Work out the finished part from the listing and answer in its coordinate system (mm). Coordinates: 2 decimals unless noted, no trailing zeros. Loops run counter-clockwise (first coordinate to the right, second up) from the corner with the lowest first, then second, coordinate; pieces in that order, holes last. Notation, with made-up numbers: (59, 63) -> (65, 63) arc R19 cw to (65, 69) -> close; hole circle Ø9 at (-0.75, 3). An arc over 180 degrees is marked (long way). One line per question, with ' | ' between items.
```python
from build123d import *

# Parameters (mm, degrees)
SKETCH_1_R      = 1.5
SKETCH_1_R_2    = 1.785756588
SKETCH_1_R_3    = 1.689732538
EXTRUDE_1_DEPTH = 6


with BuildPart() as part:
    # 草图1 → 凸台-拉伸1 (new body)
    # profile 1 of 2: a face of its own
    with BuildSketch(Plane(origin=(0, 0, 0), x_dir=(0, 0, -1), z_dir=(1, 0, 0))):
        with BuildLine():
            ThreePointArc((-172.5, 0), (0, -172.5), (172.5, 0))
            Line((172.5, 0), (-41.730591699, 0))
            Line((-41.730591699, 0), (-41.730591699, -2))
            ThreePointArc((-41.730591699, -2), (-42.023484918, -2.707106781), (-42.730591699, -3))
            Line((-42.730591699, -3), (-80.730591699, -3))
            ThreePointArc((-80.730591699, -3), (-81.43769848, -2.707106781), (-81.730591699, -2))
            Line((-81.730591699, -2), (-81.730591699, 0))
            Line((-81.730591699, 0), (-172.5, 0))
        make_face()
        with Locations((-138.564064605, -80)):
            Circle(SKETCH_1_R, mode=Mode.SUBTRACT)
        with Locations((-15, -56.936329309)):
            Circle(SKETCH_1_R_2, mode=Mode.SUBTRACT)
        with Locations((-15, -32.936329309)):
            Circle(SKETCH_1_R_2, mode=Mode.SUBTRACT)
        with Locations((0, -160)):
            Circle(SKETCH_1_R, mode=Mode.SUBTRACT)
        with Locations((15, -56.936329309)):
            Circle(SKETCH_1_R_2, mode=Mode.SUBTRACT)
        with Locations((15, -32.936329309)):
            Circle(SKETCH_1_R_2, mode=Mode.SUBTRACT)
        with Locations((138.564064606, -80)):
            Circle(SKETCH_1_R, mode=Mode.SUBTRACT)
    # profile 2 of 2: a face of its own
    with BuildSketch(Plane(origin=(0, 0, 0), x_dir=(0, 0, -1), z_dir=(1, 0, 0))):
        with BuildLine():
            Line((-41.730591699, 0), (172.5, 0))
            ThreePointArc((172.5, 0), (0, 172.5), (-172.5, 0))
            Line((-172.5, 0), (-81.730591699, 0))
            Line((-81.730591699, 0), (-81.730591699, 2))
            ThreePointArc((-81.730591699, 2), (-81.43769848, 2.707106781), (-80.730591699, 3))
            Line((-80.730591699, 3), (-42.730591699, 3))
            ThreePointArc((-42.730591699, 3), (-42.023484918, 2.707106781), (-41.730591699, 2))
            Line((-41.730591699, 2), (-41.730591699, 0))
        make_face()
        with Locations((-138.564064605, 80)):
            Circle(SKETCH_1_R, mode=Mode.SUBTRACT)
        with Locations((-15, 32.936329309)):
            Circle(SKETCH_1_R_3, mode=Mode.SUBTRACT)
        with Locations((-15, 56.936329309)):
            Circle(SKETCH_1_R_3, mode=Mode.SUBTRACT)
        with Locations((0, 160)):
            Circle(SKETCH_1_R, mode=Mode.SUBTRACT)
        with Locations((15, 32.936329309)):
            Circle(SKETCH_1_R_3, mode=Mode.SUBTRACT)
        with Locations((15, 56.936329309)):
            Circle(SKETCH_1_R_3, mode=Mode.SUBTRACT)
        with Locations((138.564064606, 80)):
            Circle(SKETCH_1_R, mode=Mode.SUBTRACT)
    extrude(amount=-EXTRUDE_1_DEPTH)


solid = part.part
```
1) Find the intervals of material crossed by line 1 along Y through (x, z) = (-2.65, 0); line 2 along Z through (x, y) = (-1.7, -80); line 3 along Y through (x, z) = (-5.05, -1), in increasing order.
Check values:
line 1: y = -172.5 to -161.5, -158.5 to 158.5, 161.5 to 172.5 | line 2: z = -152.83 to -140.06, -137.06 to 137.06, 140.06 to 152.83 | line 3: y = -172.5 to -161.12, -158.88 to 158.88, 161.12 to 172.5
2) Flat-ended cylindrical pins translate along their axes: pin 1 (4 mm diameter, centred on y = 56.94, z = -15, fed in from +X); pin 2 (2 mm diameter, centred on x = -1.5, z = -41, fed in from +Y); pin 3 (1 mm diameter, centred on x = -5.5, z = -3, fed in from +Y); pin 4 (2 mm diameter, centred on x = -3, z = -50, fed in from +Y). Find the tip coordinate at first contact, or state that the pin passes through.
Check values:
pin 1: stops at x = 0 | pin 2: stops at y = 167.8 | pin 3: stops at y = 172.48 | pin 4: stops at y = 165.39
3) Find section D-D (z = -56). Write down the section's boundary in (x, y).
Check values:
outline: (-6, -163.16) -> (0, -163.16) -> (0, 163.16) -> (-6, 163.16) -> close
4) Find section C-C (y = -138). Write down the section's boundary in (x, z).
Check values:
outline: (-6, -103.5) -> (0, -103.5) -> (0, 103.5) -> (-6, 103.5) -> close
5) Find section B-B (x = -4.65). State how many separate pieces and enclosed holes the cut face has, plus the area to 3 significant figures.
Check values:
separate pieces: 1 | enclosed holes: 15 | area: 93,100 mm^2
6) Find section A-A (z = 67). Write down the section's boundary in (x, y).
Check values:
outline: (-6, -158.96) -> (0, -158.96) -> (0, -3) -> (-6, -3) -> close; (-6, 3) -> (0, 3) -> (0, 158.96) -> (-6, 158.96) -> close
